The model under review builds one solid part; all positions refer to its coordinate system, in mm. Give positions to 0.01 mm unless a question says otherwise; leave off trailing zeros. Loops run counter-clockwise (first coordinate to the right, second up) from the corner with the lowest first, then second, coordinate; pieces in that order, holes last. Notation, with made-up numbers: M 61.25,8 L 98.25,8 A12 ccw 98.25,18 Z; hole C 44,45.25 d6. An arc over 180 degrees is marked long. One line per item, written item: value. Start each with the question number.
Q1. We need section B-B on y = 1.3. Write out the cut boundary in (x, z).
Q2. We need section A-A on x = 198.5. Write out the cut boundary in (y, z), plus the area to 3 significant figures.
Q3. To check wall thickness, follow line 1 along X through (y, z) = (0.9, -51); line 2 along Z through (x, y) = (50.5, 2.4). State the ranges of each line that lie inside material, in increasing order. Write a range as from..to.
```python
from build123d import *

# Parameters (mm, degrees)
SKETCH1_W           = 303
SKETCH1_H           = 130
BOSS_EXTRUDE1_DEPTH = 2.73


with BuildPart() as part:
    # Sketch1 → Boss-Extrude1 (new body)
    with BuildSketch(Plane(origin=(0, 0, 0), x_dir=(1, 0, 0), z_dir=(0, 1, 0))):
        with Locations((151.5, 20.018589385)):
            Rectangle(SKETCH1_W, SKETCH1_H)
        with BuildLine():
            Line((31.667883176, -31.951410615), (59.962116824, -31.951410615))
            ThreePointArc((59.962116824, -31.951410615), (63.07, -27.876410615), (59.962116824, -23.801410615))
            Line((59.962116824, -23.801410615), (31.667883176, -23.801410615))
            ThreePointArc((31.667883176, -23.801410615), (28.56, -27.876410615), (31.667883176, -31.951410615))
        make_face(mode=Mode.SUBTRACT)
        with BuildLine():
            Line((191.162705572, 55.23720125), (219.45693922, 55.23720125))
            ThreePointArc((219.45693922, 55.23720125), (222.564822396, 51.16220125), (219.45693922, 47.08720125))
            Line((219.45693922, 47.08720125), (191.162705572, 47.08720125))
            ThreePointArc((191.162705572, 47.08720125), (188.054822396, 51.16220125), (191.162705572, 55.23720125))
        make_face(mode=Mode.SUBTRACT)
        with BuildLine():
            Line((31.667883176, 47.08720125), (59.962116824, 47.08720125))
            ThreePointArc((59.962116824, 47.08720125), (63.07, 51.16220125), (59.962116824, 55.23720125))
            Line((59.962116824, 55.23720125), (31.667883176, 55.23720125))
            ThreePointArc((31.667883176, 55.23720125), (28.56, 51.16220125), (31.667883176, 47.08720125))
        make_face(mode=Mode.SUBTRACT)
        with BuildLine():
            Line((191.162705572, -31.951410615), (219.45693922, -31.951410615))
            ThreePointArc((219.45693922, -31.951410615), (222.564822396, -27.876410615), (219.45693922, -23.801410615))
            Line((219.45693922, -23.801410615), (191.162705572, -23.801410615))
            ThreePointArc((191.162705572, -23.801410615), (188.054822396, -27.876410615), (191.162705572, -31.951410615))
        make_face(mode=Mode.SUBTRACT)
    extrude(amount=BOSS_EXTRUDE1_DEPTH)


solid = part.part
```
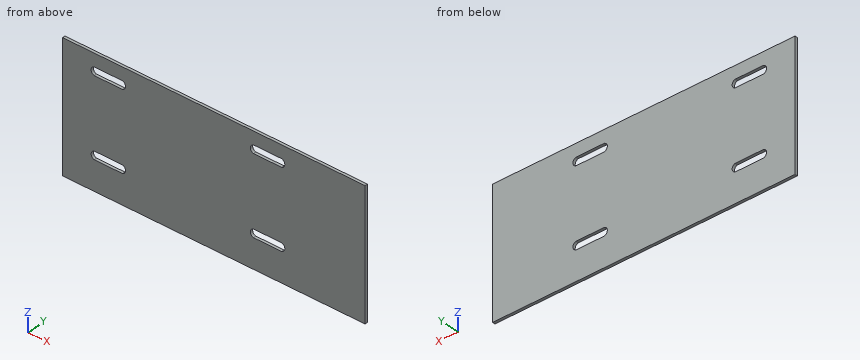
Solved:
1. outline: M 0,-85.02 L 303,-85.02 L 303,44.98 L 0,44.98 Z; hole M 31.67,-55.24 L 59.96,-55.24 A4.23 ccw 59.96,-47.09 L 31.67,-47.09 A4.23 ccw Z; hole M 31.67,23.8 L 59.96,23.8 A4.23 ccw 59.96,31.95 L 31.67,31.95 A4.23 ccw Z; hole M 191.16,-55.24 L 219.46,-55.24 A4.23 ccw 219.46,-47.09 L 191.16,-47.09 A4.23 ccw Z; hole M 191.16,23.8 L 219.46,23.8 A4.23 ccw 219.46,31.95 L 191.16,31.95 A4.23 ccw Z
2. outline: M 0,-85.02 L 2.73,-85.02 L 2.73,-55.24 L 0,-55.24 Z; M 0,-47.09 L 2.73,-47.09 L 2.73,23.8 L 0,23.8 Z; M 0,31.95 L 2.73,31.95 L 2.73,44.98 L 0,44.98 Z
2. area: 310 mm2
3. line 1: 0..28.56, 63.07..188.06, 222.56..303
3. line 2: -85.02..-55.24, -47.09..23.8, 31.95..44.98
